Work out the finished part from the listing and answer in its coordinate system (mm). Face numbers are marked on the shaded views. A direction names the side the tool comes from. Round coordinates to 2 decimals unless told otherwise and drop trailing zeros. Write each loop counter-clockwise with the first axis right and the second up, starting at its lowest first coordinate (ties: lowest second). Pieces come first, ordered by that corner, then holes. Notation, with made-up numbers: (-40, -23) - (19, -23) arc R22 cw to (19, 0) - close; hole circle Ø10 at (29.5, -34.75). An arc over 180 degrees is marked (long way). Answer as a JSON object with one key per item and string values.
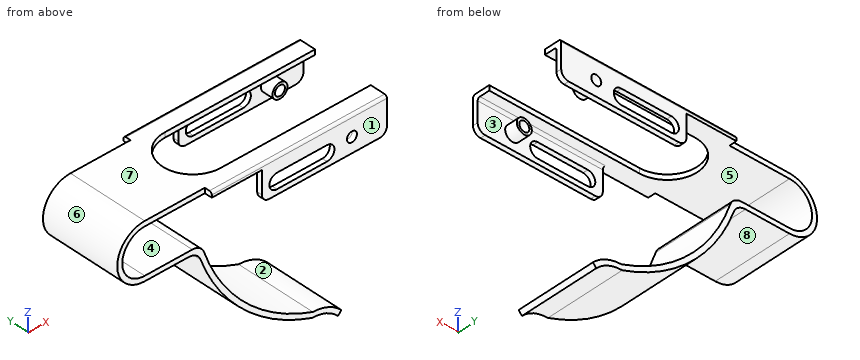
```python
from build123d import *

# Parameters (mm, degrees)
F1_DEPTH  = 16
F2_W      = 70
F2_H      = 3
F3_DEPTH  = 2
F4_W      = 50
F4_H      = 14
F5_DEPTH  = 2
F6_R      = 1
F9_DEPTH  = 2
F11_DEPTH = 38.001
F13_D     = 4
F14_R     = 3
F14_R_2   = 2
F15_DEPTH = 5
F16_R     = 3


# Not quite as in the source:
# - a pattern or mirror of a feature is missing from the dataset's text; its kind, count and spacing are read off the source's solid


with BuildPart() as f1:
    # F0 (on Front) → F1 (new body)
    with BuildSketch(Plane.XZ):
        with BuildLine():
            Line((94, 11), (0, 11))
            ThreePointArc((0, 11), (-11, 0), (0, -11))
            Line((0, -11), (17.5822146692, -11))
            ThreePointArc((17.5822146692, -11), (20.4548889983, -11.9075994576), (22.2846682622, -14.3009031203))
            ThreePointArc((22.2846682622, -14.3009031203), (39.5706846565, -41.223441559), (66.8144425174, -57.9986344457))
            ThreePointArc((66.8144425174, -57.9986344457), (72.5102657096, -59.1645299936), (77.2413235191, -62.5437024171))
            Line((77.2413235191, -62.5437024171), (78.536643648, -61))
            ThreePointArc((78.536643648, -61), (73.3497255449, -57.3487659198), (67.1516242057, -56))
            ThreePointArc((67.1516242057, -56), (40.3930033582, -39.2216179023), (23.7333333333, -12.3889272035))
            ThreePointArc((23.7333333333, -12.3889272035), (21.9107246536, -9.9345748081), (19, -9))
            Line((19, -9), (0, -9))
            ThreePointArc((0, -9), (-9, 0), (0, 9))
            Line((0, 9), (94, 9))
            Line((94, 9), (94, 11))
        make_face()
    extrude(amount=F1_DEPTH)

    # F2 (on face) → F3 (join)
    with BuildSketch(Plane.XY.offset(11)):
        with Locations((59, -17.5)):
            Rectangle(F2_W, F2_H)
    extrude(amount=-F3_DEPTH)

    # F4 (on face) → F5 (join)
    with BuildSketch(Plane.XZ.offset(19)):
        with Locations((69, 4)):
            Rectangle(F4_W, F4_H)
    extrude(amount=-F5_DEPTH)

    # F6
    f6_edges = [f1.edges().sort_by_distance(p)[0] for p in [
        (59, -19, 11),
        (69, -17, 9),
    ]]
    fillet(f6_edges, radius=F6_R)

    # F7: F1 across plane


with BuildPart() as f1_1:
    add(f1.part)
    add(f1.part.mirror(Plane.XZ))

    # F8 (on face) → F9 (cut)
    with BuildSketch(Plane.XY.offset(11)):
        with BuildLine():
            Line((94, 12), (34, 12))
            ThreePointArc((34, 12), (22, 0), (34, -12))
            Line((34, -12), (94, -12))
            Line((94, -12), (94, 12))
        make_face()
    extrude(amount=-F9_DEPTH, mode=Mode.SUBTRACT)

    # F10 (on face) → F11 (cut, through all)
    with BuildSketch(Plane.XZ.offset(19)):
        with BuildLine():
            ThreePointArc((50, 5), (47, 2), (50, -1))
            Line((50, -1), (70, -1))
            ThreePointArc((70, -1), (73, 2), (70, 5))
            Line((70, 5), (50, 5))
        make_face()
    extrude(amount=-F11_DEPTH, mode=Mode.SUBTRACT)

    # F13 (through all)
    with Locations(Plane.XZ.offset(19)):
        with Locations((80, 3)):
            Hole(F13_D / 2)

    # F14 (on face) → F15 (join)
    with BuildSketch(Plane(origin=(0, -17, 0), x_dir=(-1, 0, 0), z_dir=(0, 1, 0))):
        with Locations((-80, 3)):
            Circle(F14_R)
        with Locations((-80, 3)):
            Circle(F14_R_2, mode=Mode.SUBTRACT)
    f15 = extrude(amount=F15_DEPTH)

    # F15_copies: F15 across plane
    add(f15.mirror(Plane.ZX))

    # F16
    f16_edges = [f1_1.edges().sort_by_distance(p)[0] for p in [
        (44, -18, -3),
        (94, -18, -3),
        (44, 18, -3),
        (94, 18, -3),
    ]]
    fillet(f16_edges, radius=F16_R)


solid = f1_1.part
```
Item 1: Each of these flat-tipped pins is pushed along its axis until it touches: P1, Ø2, axis at x = 71.5, y = 17.5, coming from the -Z side; P2, Ø3.5, axis at x = 80, z = 3, coming from the -Y side; P3, Ø3.5, axis at y = 18, z = 2.5, coming from the -X side; P4, Ø2, axis at y = 14, z = -12.5, coming from the -X side. Where does it stop, or does it pass through?
Results found:
{"P1": "z = -3", "P2": "through", "P3": "x = 44", "P4": "x = 19.76"}
Item 2: For the marked faces 4, 5, 6, 7 and 8, determine the directions among +Z, -Z, +X, -X, +Y, -Y from which every point of the face is accessible in a straight line to the end or side of a thin tool.
Results found:
{"face 4": "+X, +Y, -Y", "face 5": "none", "face 6": "-X, +Y, -Y", "face 7": "+Z, +X, -X, +Y, -Y", "face 8": "-Z, -X, +Y, -Y"}
Item 3: Consider line 1 along Z through (x, y) = (80, -14.3); line 2 along Z through (x, y) = (36, -2.5); line 3 along Z through (x, y) = (68.5, -14.5). Determine where each line is inside the solid, lowest interval first.
Results found:
{"line 1": "0 to 1, 5 to 6, 9 to 11", "line 2": "-37.46 to -34.38", "line 3": "-58.09 to -56.08, 9 to 11"}
Item 4: A cutting plane is placed at C-C (x = 53.5). Write down the section's boundary in (y, z).
Results found:
{"outline": "(-19, -3) - (-17, -3) - (-17, -1) - (-19, -1) - close; (-19, 5) - (-17, 5) - (-17, 8) arc R1 cw to (-16, 9) - (-12, 9) - (-12, 11) - (-18, 11) arc R1 ccw to (-19, 10) - close; (-16, -51.9) - (16, -51.9) - (16, -49.56) - (-16, -49.56) - close; (12, 9) - (16, 9) arc R1 cw to (17, 8) - (17, 5) - (19, 5) - (19, 10) arc R1 ccw to (18, 11) - (12, 11) - close; (17, -3) - (19, -3) - (19, -1) - (17, -1) - close"}
Item 5: Determine the mould class of the marked faces 1, 2 and 3 for opening direction Y: pulls with the +Y half, pulls with the -Y half, needs draft (parallel to the pull), parting line crosses it, or undercut.
Results found:
{"face 1": "pulls with the -Y half", "face 2": "needs draft", "face 3": "undercut"}
Item 6: A cutting plane is placed at D-D (z = 3). Give the number of separate pieces and of enclosed holes in the cut face, and give its area (4 significant figures).
Results found:
{"separate pieces": "7", "enclosed holes": "0", "area": "168.5 mm²"}
Item 7: A cutting plane is placed at A-A (x = 39.5). Write down the section's boundary in (y, z), and give its area (3 significant figures).
Results found:
{"outline": "(-19, 9) - (-12, 9) - (-12, 11) - (-18, 11) arc R1 ccw to (-19, 10) - close; (-16, -41.15) - (16, -41.15) - (16, -38.31) - (-16, -38.31) - close; (12, 9) - (19, 9) - (19, 10) arc R1 ccw to (18, 11) - (12, 11) - close", "area": "119 mm²"}
Item 8: A cutting plane is placed at B-B (y = 0). Write down the section's boundary in (x, z).
Results found:
{"outline": "(0, -11) - (17.58, -11) arc R5 cw to (22.28, -14.3) arc R72 ccw to (66.81, -58) arc R14 cw to (77.24, -62.54) - (78.54, -61) arc R16 ccw to (67.15, -56) arc R70 cw to (23.73, -12.39) arc R5 ccw to (19, -9) - (0, -9) arc R9 cw to (0, 9) - (22, 9) - (22, 11) - (0, 11) arc R11 ccw to start"}
